from build123d import *

# Parameters (mm, degrees)
SKETCH1_R             = 146
SKETCH1_R_2           = 50.8
BOSS_EXTRUDE1_DEPTH   = 3.175
F_4_CLEARANCE_HOLE1_D = 3.2639
CIRPATTERN1_COUNT     = 10


with BuildPart() as part:
    # Sketch1 → Boss-Extrude1 (new body)
    with BuildSketch(Plane.XY):
        Circle(SKETCH1_R)
        Circle(SKETCH1_R_2, mode=Mode.SUBTRACT)
    extrude(amount=BOSS_EXTRUDE1_DEPTH)

    # #4 Clearance Hole1 (through all)
    with Locations(Plane.XY.offset(3.175)):
        with Locations((0, 142)):
            f_4_clearance_hole1 = Hole(F_4_CLEARANCE_HOLE1_D / 2)

    # CirPattern1: #4 Clearance Hole1 ×10 about axis
    cirpattern1_axis = Axis((0, 0, 0), (0, 0, 1))
    for i in range(1, CIRPATTERN1_COUNT):
        add(f_4_clearance_hole1.rotate(cirpattern1_axis, i * 360 / CIRPATTERN1_COUNT), mode=Mode.SUBTRACT)


solid = part.part
For this review, take the finished solid that the model builds, in its own axes (mm). Round coordinates to 2 decimals unless told otherwise and drop trailing zeros. Loops run counter-clockwise (first coordinate to the right, second up) from the corner with the lowest first, then second, coordinate; pieces in that order, holes last. Notation, with made-up numbers: (12, -20.75) - (61, -20.75) arc R28 cw to (61, 8.25) - close; hole circle Ø6 at (39, 9.25). An arc over 180 degrees is marked (long way). Answer as CSV lines item,"result".
(1) Wall thickness on line 1 (Y direction, x = 11.5, z = 2.95); line 2 (Y direction, x = -32, z = 2.15); line 3 (X direction, y = -16.5, z = 2.1): over which ranges is each line inside the solid? List them lowest first.
Checked values:
line 1,"y = -145.55 to -49.48, 49.48 to 145.55"
line 2,"y = -142.45 to -39.45, 39.45 to 142.45"
line 3,"x = -145.06 to -48.05, 48.05 to 145.06"
(2) Consider section B-B on z = 1.25. Give the number of separate pieces and of enclosed holes in the cut face, then the cut area to 3 significant figures.
Checked values:
separate pieces,"1"
enclosed holes,"11"
area,"58,800 mm2"
(3) Consider section D-D on x = -125. Give the boundary of the cut face in (y, z) (3 decimals), then the cut area to 3 significant figures.
Checked values:
outline,"(-75.439, 0) - (75.439, 0) - (75.439, 3.175) - (-75.439, 3.175) - close"
area,"479 mm2"
(4) Consider section C-C on x = -16. Give the boundary of the cut face in (y, z) (3 decimals).
Checked values:
outline,"(-145.121, 0) - (-48.215, 0) - (-48.215, 3.175) - (-145.121, 3.175) - close; (48.215, 0) - (145.121, 0) - (145.121, 3.175) - (48.215, 3.175) - close"
(5) Consider section A-A on y = 0. Give the boundary of the cut face in (x, z) (3 decimals), then the cut area to 3 significant figures.
Checked values:
outline,"(-146, 0) - (-50.8, 0) - (-50.8, 3.175) - (-146, 3.175) - close; (50.8, 0) - (146, 0) - (146, 3.175) - (50.8, 3.175) - close"
area,"605 mm2"
(6) Mouldability with a two-part tool opening along X and no side actions: class faces 1 (the face through (-31.65, -142.53, 1.57)), 2 (the face through (-11.012, -49.592, 1.565)), 3 (the face through (63, 2, 3.175)) as +X half, -X half, draft (parallel to the pull), parting line (faces both ways), or undercut.
Checked values:
face 1,"parting line"
face 2,"undercut"
face 3,"draft"
